Input: dimensioned drawing with shaded views. Units: mm. Origin: part minimum x, y, z. Give positions to 0.01 mm unless a question says otherwise; leave off trailing zeros. Answer in a Markdown table with one row per item.
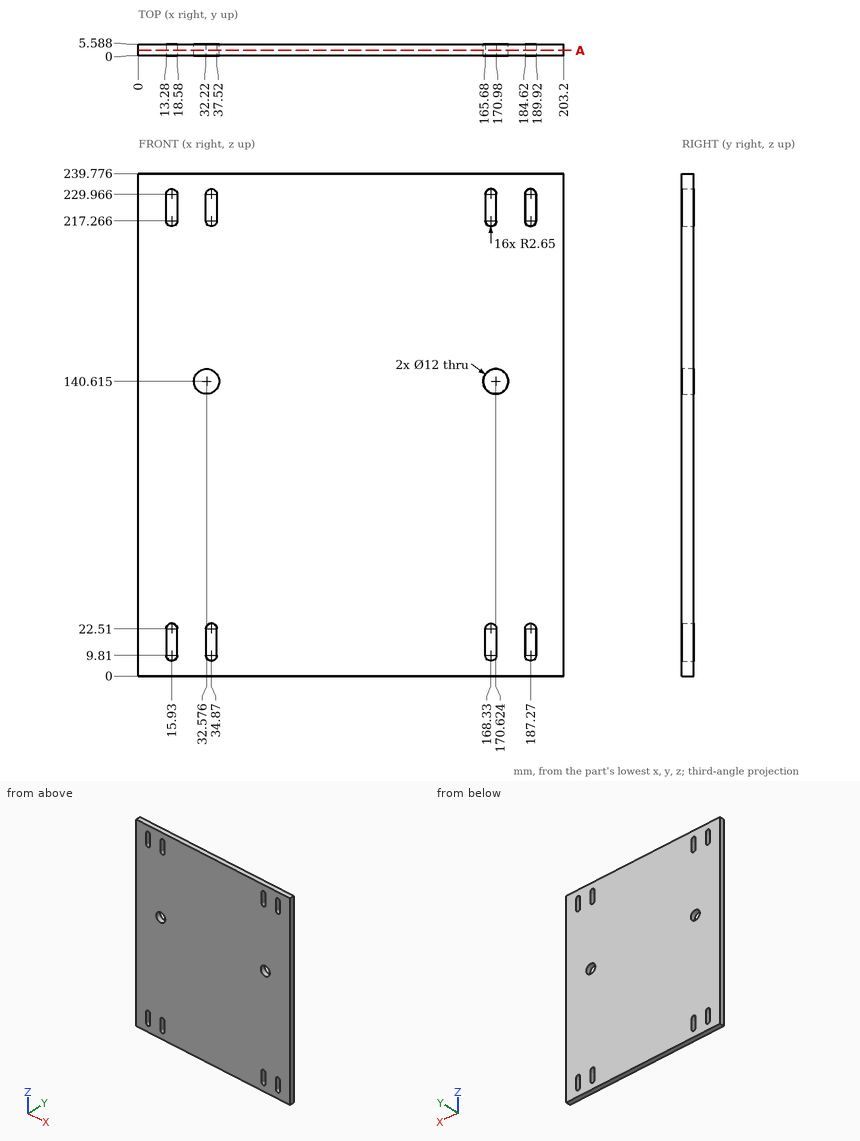
Q1. Ray query, probe 1 along X at (y, z) = (3.4, 220.5); probe 2 along Z at (x, y) = (30, 2.05) (1 decimal). Return the intervals inside material, ascending. Write a range as from..to.
Values follow:
| item | result |
|---|---|
| probe 1 | 0..13.28, 18.58..32.22, 37.52..165.68, 170.98..184.62, 189.92..203.2 |
| probe 2 | 0..135.2, 146..239.8 |
Q2. Contact query for a flat-ended pin moving along its axis: pin 1 Ø3 at (y, z) = (4, 152) entering from -X. Output: stop coordinate, or through.
Values follow:
| item | result |
|---|---|
| pin 1 | x = 0 |
Q3. Section query A-A (y = 2.55). Give the number of separate pieces and of enclosed holes in the cut face, plus the area to 3 significant figures.
Values follow:
| item | result |
|---|---|
| separate pieces | 1 |
| enclosed holes | 10 |
| area | 47,800 mm^2 |
